Drawing for the job (mm, zero at the part's lowest x, y, z). A direction names the side the tool comes from. Round coordinates to 2 decimals unless told otherwise and drop trailing zeros. Write each loop counter-clockwise with the first axis right and the second up, starting at its lowest first coordinate (ties: lowest second). Pieces come first, ordered by that corner, then holes. Notation, with made-up numbers: (-15, 62) -> (19, 62) arc R10 ccw to (19, 69) -> close; hole circle Ø5 at (1.25, 14). An arc over 180 degrees is marked (long way). Answer in a Markdown table with one row per item. Add a question column.
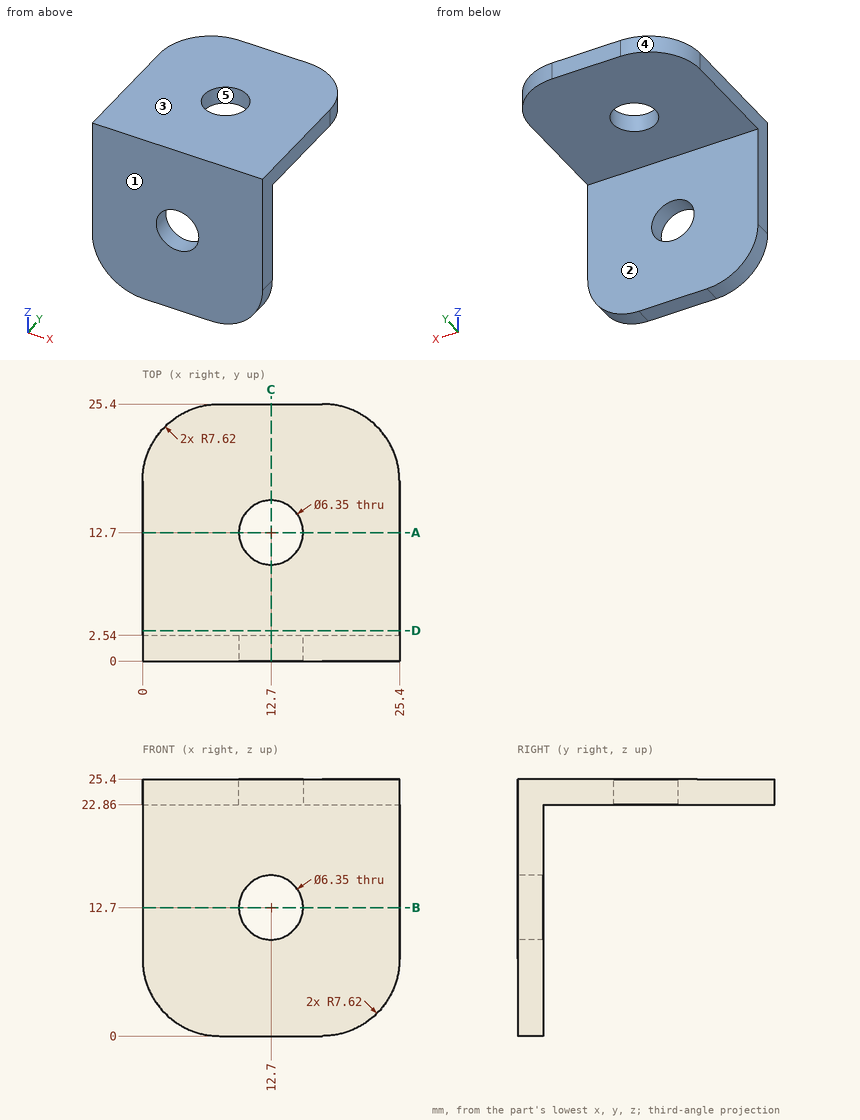
(1) Probe line 1 along Y through (x, z) = (12.7, 24.1) (3 decimals); line 2 along Z through (x, y) = (7.75, 6.25). List the from-to ranges inside material, lowest first.
(2) Saw through at B-B (z = 12.7). List the corners of the cut face in (x, y) (3 decimals), plus the area to 3 significant figures.
(3) Saw through at C-C (x = 12.7). List the corners of the cut face in (y, z) (3 decimals).
(4) Saw through at A-A (y = 12.7). List the corners of the cut face in (x, z) (3 decimals).
(5) Drop flat-ended pins along their axis: P1, Ø1.5, axis at x = 18, z = 4.5, coming from the +Y side; P2, Ø8, axis at x = 3, z = 15.5, coming from the -Y side; P3, Ø5, axis at x = 12.7, z = 12.7, coming from the +Y side; P4, Ø1, axis at x = 14, y = 10, coming from the -Z side. Give the stop position or say it passes through.
(6) Which spindle directions (+Z, -Z, +X, -X, +Y, -Y) get a long thin tool onto all of the face, cutting with end or side? Do the marked faces 1 and 2. Say none if no direction does.
(7) Saw through at D-D (y = 3). List the corners of the cut face in (x, z).
(8) Mould opens along X. For the marked faces 3, 4 and 5 say: pulls with the +X half, pulls with the -X half, needs draft (parallel to the pull), parting line crosses it, or undercut.
Answer sheet:
| question | item | result |
|---|---|---|
| 1 | line 1 | y = 0 to 9.525, 15.875 to 25.4 |
| 1 | line 2 | z = 22.86 to 25.4 |
| 2 | outline | (0, 0) -> (9.525, 0) -> (9.525, 2.54) -> (0, 2.54) -> close; (15.875, 0) -> (25.4, 0) -> (25.4, 2.54) -> (15.875, 2.54) -> close |
| 2 | area | 48.4 mm² |
| 3 | outline | (0, 0) -> (2.54, 0) -> (2.54, 9.525) -> (0, 9.525) -> close; (0, 15.875) -> (2.54, 15.875) -> (2.54, 22.86) -> (9.525, 22.86) -> (9.525, 25.4) -> (0, 25.4) -> close; (15.875, 22.86) -> (25.4, 22.86) -> (25.4, 25.4) -> (15.875, 25.4) -> close |
| 4 | outline | (0, 22.86) -> (9.525, 22.86) -> (9.525, 25.4) -> (0, 25.4) -> close; (15.875, 22.86) -> (25.4, 22.86) -> (25.4, 25.4) -> (15.875, 25.4) -> close |
| 5 | P1 | stops at y = 2.54 |
| 5 | P2 | stops at y = 0 |
| 5 | P3 | passes through |
| 5 | P4 | stops at z = 22.86 |
| 6 | face 1 | +Z, -Z, +X, -X, -Y |
| 6 | face 2 | -Z, +X, -X, +Y |
| 7 | outline | (0, 22.86) -> (25.4, 22.86) -> (25.4, 25.4) -> (0, 25.4) -> close |
| 8 | face 3 | needs draft |
| 8 | face 4 | pulls with the -X half |
| 8 | face 5 | undercut |
